from build123d import *

# Parameters (mm, degrees)
SKETCH1_R           = 8.001
BOSS_EXTRUDE1_DEPTH = 44.45
SKETCH2_R           = 7.62
CUT_EXTRUDE1_DEPTH  = 43.18
SKETCH3_R           = 6.35
CUT_EXTRUDE2_DEPTH  = 1.27
CHAMFER2_SIZE       = 1.27


with BuildPart() as part:
    # Sketch1 → Boss-Extrude1 (new body)
    with BuildSketch(Plane(origin=(0, 0, 0), x_dir=(1, 0, 0), z_dir=(0, 1, 0))):
        with Locations(Location((0, 0, 0), (0, 0, 270))):
            Circle(SKETCH1_R)
    extrude(amount=BOSS_EXTRUDE1_DEPTH)

    # Sketch2 → Cut-Extrude1 (cut)
    with BuildSketch(Plane(origin=(0, 44.45, 0), x_dir=(1, 0, 0), z_dir=(0, 1, 0))):
        with Locations(Location((0, 0, 0), (0, 0, 270))):
            Circle(SKETCH2_R)
    extrude(amount=-CUT_EXTRUDE1_DEPTH, mode=Mode.SUBTRACT)

    # Sketch3 → Cut-Extrude2 (cut)
    with BuildSketch(Plane(origin=(0, 1.27, 0), x_dir=(1, 0, 0), z_dir=(0, 1, 0))):
        with Locations(Location((0, 0, 0), (0, 0, 270))):
            Circle(SKETCH3_R)
    extrude(amount=-CUT_EXTRUDE2_DEPTH, mode=Mode.SUBTRACT)

    # Chamfer2
    chamfer2_edges = [part.edges().sort_by_distance(p)[0] for p in [
        (0, 0, -6.35),
    ]]
    chamfer(chamfer2_edges, length=CHAMFER2_SIZE - 0.0001)  # a hair under: the kernel refuses the full size

    # Sketch5 → Revolve1 (revolve)
    with BuildSketch(Plane.XY, mode=Mode.PRIVATE) as revolve1_sk:
        with BuildLine():
            Line((8.001, 44.45), (13.698005601, 44.45))
            Line((13.698005601, 44.45), (13.698005601, 41.91))
            ThreePointArc((13.698005601, 41.91), (10.812623084, 41.67859503), (8.001, 40.990295557))
            Line((8.001, 40.990295557), (8.001, 44.45))
        make_face()
    revolve(revolve1_sk.sketch.rotate(Axis((0, 1.27, 0), (0, 1, 0)), 90), axis=Axis((0, 1.27, 0), (0, 1, 0)))


solid = part.part
Verification items for the finished model (mm, model axes). A direction names the side the tool comes from. Coordinates: 2 decimals unless noted, no trailing zeros. Write each loop counter-clockwise with the first axis right and the second up, starting at its lowest first coordinate (ties: lowest second). Pieces come first, ordered by that corner, then holes. Notation, with made-up numbers: (7, 15) -> (17, 15) arc R15 ccw to (17, 27) -> close; hole circle Ø6 at (81, -29). An arc over 180 degrees is marked (long way). One line per item, written item: value. Start each with the question number.
Q1. Cross-section at A-A on y = 39. Enter the section's corners in (x, z).
Q2. Access from +Z, -Z, +X, -X, +Y, -Y to the whole of each face (thin tool, end or side, straight path). Record for faces 1 (the cylindrical face through (2.403, 20.208, 7.632)), 2 (the cylindrical face through (7.555, 23.162, -0.992)).
Q3. Thickness scan on L1, parallel to X at y = 1.35, z = 0; L2, parallel to X at y = 26.5, z = 3.25; L3, parallel to Z at x = -2.5, y = 20. Record the ranges inside material, lowest first. Write a range as from..to.
Q4. Go/stop test with flat-tipped pins: P1, Ø7.5, axis at x = -2.5, z = -1.5, coming from the +Y side; P2, Ø1, axis at x = 7.5, y = 33, coming from the -Z side; P3, Ø5, axis at y = 38, z = 5, coming from the +X side. Record where each tip stops, or that it passes through.
Q5. Mould release check, pull along Z, two halves, no side actions. Record for faces 3 (the cylindrical face through (12.152, 43.162, -6.321)), 4 (the flat face through (6, 1.27, -3)), 5 (the flat face through (6, 44.45, 6)): pulls with the +Z half, pulls with the -Z half, needs draft (parallel to the pull), parting line crosses it, or undercut.
Checked values:
1. outline: circle Ø16 at (0, 0); hole circle Ø15.24 at (0, 0)
2. face 1: -Y
2. face 2: +Y
3. L1: x = -8..-7.62, 7.62..8
3. L2: x = -7.31..-6.89, 6.89..7.31
3. L3: z = -7.6..-7.2, 7.2..7.6
4. P1: stops at y = 1.27
4. P2: stops at z = -3.88
4. P3: stops at x = 7.6
5. face 3: parting line crosses it
5. face 4: undercut
5. face 5: needs draft
